Check sheet for the drawn part. Datum: minimum x, y, z corner. Units: mm. Coordinates: 2 decimals unless noted, no trailing zeros. Order: outer loops, then holes, each group sorted by start corner. A loop starts at its lowest first (then second) coordinate and runs counter-clockwise, first axis right, second up. Notation, with made-up numbers: (78.25, 68) - (82.25, 68) arc R31 ccw to (82.25, 96) - close; hole circle Ø3 at (76.25, -31.75). An arc over 180 degrees is marked (long way). Answer as CSV lines item,"result". Start each with the question number.
1. Go/stop test with a flat-tipped pin: pin 1 (0.8 mm diameter, centred on x = 29, z = 1, fed in from +Y). Record where the tip stops, or that it passes through.
2. Section check A-A (y = 11). Record the cut outline in (x, z).
3. Section check C-C (z = 1). Record the cut outline in (x, y), and give its area (3 significant figures).
4. Section check D-D (x = 87.25). Record the cut outline in (y, z), and give its area (4 significant figures).
5. Material ranges on L1, parallel to X at y = 21.25, z = 1.2; L2, parallel to X at y = 9.75, z = 0.15; L3, parallel to Y at x = 15, z = 1, recorded low to high. Write a range as [from, to].
6. Section check B-B (x = 15). Record the cut outline in (y, z).
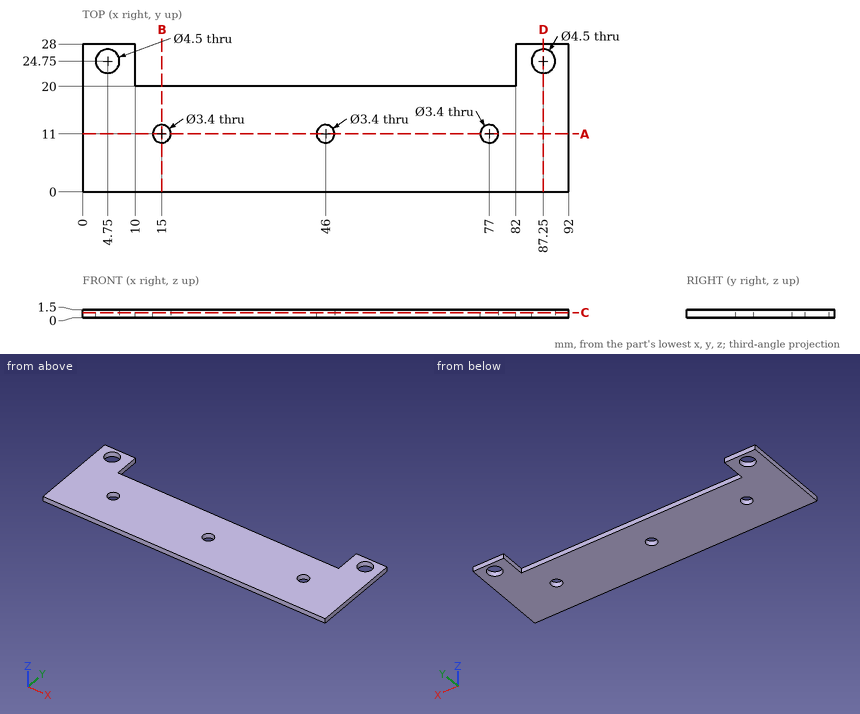
Evaluation:
1,pin 1,"stops at y = 20"
2,outline,"(0, 0) - (13.3, 0) - (13.3, 1.5) - (0, 1.5) - close; (16.7, 0) - (44.3, 0) - (44.3, 1.5) - (16.7, 1.5) - close; (47.7, 0) - (75.3, 0) - (75.3, 1.5) - (47.7, 1.5) - close; (78.7, 0) - (92, 0) - (92, 1.5) - (78.7, 1.5) - close"
3,outline,"(0, 0) - (92, 0) - (92, 28) - (82, 28) - (82, 20) - (10, 20) - (10, 28) - (0, 28) - close; hole circle Ø4.5 at (4.75, 24.75); hole circle Ø3.4 at (15, 11); hole circle Ø3.4 at (46, 11); hole circle Ø3.4 at (77, 11); hole circle Ø4.5 at (87.25, 24.75)"
3,area,"1,940 mm²"
4,outline,"(0, 0) - (22.5, 0) - (22.5, 1.5) - (0, 1.5) - close; (27, 0) - (28, 0) - (28, 1.5) - (27, 1.5) - close"
4,area,"35.25 mm²"
5,L1,"x = [0, 10], [82, 92]"
5,L2,"x = [0, 13.85], [16.15, 44.85], [47.15, 75.85], [78.15, 92]"
5,L3,"y = [0, 9.3], [12.7, 20]"
6,outline,"(0, 0) - (9.3, 0) - (9.3, 1.5) - (0, 1.5) - close; (12.7, 0) - (20, 0) - (20, 1.5) - (12.7, 1.5) - close"
